Geometry: final body of the model. Coordinates: model frame, mm. Round coordinates to 2 decimals unless told otherwise and drop trailing zeros. Order: outer loops, then holes, each group sorted by start corner. A loop starts at its lowest first (then second) coordinate and runs counter-clockwise, first axis right, second up. Notation, with made-up numbers: M -9.5,79 L 17.5,79 A26 cw 17.5,94 Z; hole C -3.5,77 d8. An arc over 180 degrees is marked long. Return JSON: item names as keys, results as strings. Group by question number.
Q1. Cut plane B-B on x = -146. Output: boundary loops of the cut face in (y, z) (3 decimals).
Q2. Cut plane A-A on x = -36.5. Output: boundary loops of the cut face in (y, z) (3 decimals).
Q3. Cut plane C-C on z = 1. Count the separate pieces of the cut face and the enclosed holes in it, and give its area (3 significant figures).
Q4. Ray query, probe 1 along Y at (x, z) = (12, 2.9); probe 2 along Y at (x, z) = (-55.5, 2.8); probe 3 along X at (y, z) = (22.25, 0.5). Return the intervals inside material, ascending.
Q5. Contact query for a flat-ended pin moving along its axis: pin 1 (1.6 mm diameter, centred on x = -12, z = 2, fed in from +Y). Output: stop coordinate, or through.
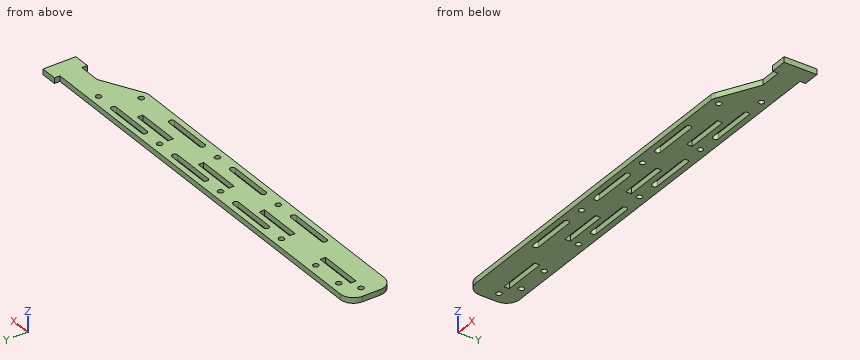
```python
from build123d import *

# Parameters (mm, degrees)
SKETCH1_R           = 1.5875
SKETCH1_W           = 25.4
SKETCH1_H           = 3.175
BOSS_EXTRUDE1_DEPTH = 3.175


with BuildPart() as part:
    # Sketch1 → Boss-Extrude1 (new body)
    with BuildSketch(Plane.XY):
        with BuildLine():
            Line((68.764710276, 20.278973895), (56.064710276, 20.278973895))
            Line((56.064710276, 20.278973895), (33.372798511, 8.176620954))
            ThreePointArc((33.372798511, 8.176620954), (32.214291251, 7.730649994), (30.982210276, 7.578973895))
            Line((30.982210276, 7.578973895), (-152.215289724, 7.578973895))
            Line((-152.215289724, 7.578973895), (-164.915289724, 7.578973895))
            ThreePointArc((-164.915289724, 7.578973895), (-170.303443397, 9.810820222), (-172.535289724, 15.198973895))
            Line((-172.535289724, 15.198973895), (-172.535289724, 23.453973895))
            Line((-172.535289724, 23.453973895), (-172.535289724, 25.358973895))
            ThreePointArc((-172.535289724, 25.358973895), (-170.303443397, 30.747127568), (-164.915289724, 32.978973895))
            Line((-164.915289724, 32.978973895), (-152.215289724, 32.978973895))
            Line((-152.215289724, 32.978973895), (68.764710276, 32.978973895))
            Line((68.764710276, 32.978973895), (68.764710276, 36.153973895))
            Line((68.764710276, 36.153973895), (78.289710276, 36.153973895))
            Line((78.289710276, 36.153973895), (78.289710276, 17.103973895))
            Line((78.289710276, 17.103973895), (68.764710276, 17.103973895))
            Line((68.764710276, 17.103973895), (68.764710276, 20.278973895))
        make_face()
        with Locations((30.664710276, 12.341473895)):
            Circle(SKETCH1_R, mode=Mode.SUBTRACT)
        with Locations((-109.035289724, 28.216473895)):
            Circle(SKETCH1_R, mode=Mode.SUBTRACT)
        with Locations((-166.185289724, 21.866473895)):
            Circle(SKETCH1_R, mode=Mode.SUBTRACT)
        with Locations((-156.660289724, 28.216473895)):
            Circle(SKETCH1_R, mode=Mode.SUBTRACT)
        with Locations((-137.610289724, 28.216473895)):
            Circle(SKETCH1_R, mode=Mode.SUBTRACT)
        with Locations((-83.635289724, 12.341473895)):
            Circle(SKETCH1_R, mode=Mode.SUBTRACT)
        with Locations((-32.835289724, 12.341473895)):
            Circle(SKETCH1_R, mode=Mode.SUBTRACT)
        with Locations((-58.235289724, 28.216473895)):
            Circle(SKETCH1_R, mode=Mode.SUBTRACT)
        with Locations((-7.435289724, 28.216473895)):
            Circle(SKETCH1_R, mode=Mode.SUBTRACT)
        with Locations((43.364710276, 28.216473895)):
            Circle(SKETCH1_R, mode=Mode.SUBTRACT)
        with Locations((-147.135289724, 21.866473895)):
            Rectangle(SKETCH1_W, SKETCH1_H, mode=Mode.SUBTRACT)
        with Locations((-96.335289724, 21.866473895)):
            Rectangle(SKETCH1_W, SKETCH1_H, mode=Mode.SUBTRACT)
        with Locations((-45.535289724, 21.866473895)):
            Rectangle(SKETCH1_W, SKETCH1_H, mode=Mode.SUBTRACT)
        with Locations((5.264710276, 21.866473895)):
            Rectangle(SKETCH1_W, SKETCH1_H, mode=Mode.SUBTRACT)
        with BuildLine():
            Line((5.264710276, 29.803973895), (30.664710276, 29.803973895))
            ThreePointArc((30.664710276, 29.803973895), (32.252210276, 28.216473895), (30.664710276, 26.628973895))
            Line((30.664710276, 26.628973895), (5.264710276, 26.628973895))
            ThreePointArc((5.264710276, 26.628973895), (3.677210276, 28.216473895), (5.264710276, 29.803973895))
        make_face(mode=Mode.SUBTRACT)
        with BuildLine():
            Line((-45.535289724, 13.928973895), (-70.935289724, 13.928973895))
            ThreePointArc((-70.935289724, 13.928973895), (-72.522789724, 12.341473895), (-70.935289724, 10.753973895))
            Line((-70.935289724, 10.753973895), (-45.535289724, 10.753973895))
            ThreePointArc((-45.535289724, 10.753973895), (-43.947789724, 12.341473895), (-45.535289724, 13.928973895))
        make_face(mode=Mode.SUBTRACT)
        with BuildLine():
            Line((-96.335289724, 13.928973895), (-121.735289724, 13.928973895))
            ThreePointArc((-121.735289724, 13.928973895), (-123.322789724, 12.341473895), (-121.735289724, 10.753973895))
            Line((-121.735289724, 10.753973895), (-96.335289724, 10.753973895))
            ThreePointArc((-96.335289724, 10.753973895), (-94.747789724, 12.341473895), (-96.335289724, 13.928973895))
        make_face(mode=Mode.SUBTRACT)
        with BuildLine():
            Line((5.264710276, 13.928973895), (-20.135289724, 13.928973895))
            ThreePointArc((-20.135289724, 13.928973895), (-21.722789724, 12.341473895), (-20.135289724, 10.753973895))
            Line((-20.135289724, 10.753973895), (5.264710276, 10.753973895))
            ThreePointArc((5.264710276, 10.753973895), (6.852210276, 12.341473895), (5.264710276, 13.928973895))
        make_face(mode=Mode.SUBTRACT)
        with BuildLine():
            Line((-45.535289724, 29.803973895), (-20.135289724, 29.803973895))
            ThreePointArc((-20.135289724, 29.803973895), (-18.547789724, 28.216473895), (-20.135289724, 26.628973895))
            Line((-20.135289724, 26.628973895), (-45.535289724, 26.628973895))
            ThreePointArc((-45.535289724, 26.628973895), (-47.122789724, 28.216473895), (-45.535289724, 29.803973895))
        make_face(mode=Mode.SUBTRACT)
        with BuildLine():
            Line((-96.335289724, 29.803973895), (-70.935289724, 29.803973895))
            ThreePointArc((-70.935289724, 29.803973895), (-69.347789724, 28.216473895), (-70.935289724, 26.628973895))
            Line((-70.935289724, 26.628973895), (-96.335289724, 26.628973895))
            ThreePointArc((-96.335289724, 26.628973895), (-97.922789724, 28.216473895), (-96.335289724, 29.803973895))
        make_face(mode=Mode.SUBTRACT)
    extrude(amount=BOSS_EXTRUDE1_DEPTH)


solid = part.part
```
Result sheet:
{
 "1": {"outline": "M 7.579,0 L 20.279,0 L 20.279,3.175 L 7.579,3.175 Z; M 23.454,0 L 32.979,0 L 32.979,3.175 L 23.454,3.175 Z"},
 "2": {"outline": "M 7.579,0 L 20.279,0 L 20.279,3.175 L 7.579,3.175 Z; M 23.454,0 L 26.629,0 L 26.629,3.175 L 23.454,3.175 Z; M 29.804,0 L 32.979,0 L 32.979,3.175 L 29.804,3.175 Z"},
 "3": {"separate pieces": "1", "enclosed holes": "20", "area": "5,040 mm²"},
 "4": {"probe 1": "y = 7.58 to 20.28, 23.45 to 26.63, 29.8 to 32.98", "probe 2": "y = 7.58 to 10.75, 13.93 to 20.28, 23.45 to 32.98", "probe 3": "x = -172.54 to -167.73, -164.64 to -159.84, -134.44 to -109.04, -83.64 to -58.24, -32.84 to -7.44, 17.96 to 78.29"},
 "5": {"pin 1": "stops at y = 32.98"}
}
